from build123d import *

# Parameters (mm, degrees)
EXTRUDE_1_DEPTH     = 40.5
SKETCH_2_R          = 1.75
CUT_EXTRUDE_1_DEPTH = 44
FILLET_6_R          = 5
SKETCH_5_R          = 3
CUT_EXTRUDE_2_DEPTH = 35
SKETCH_6_R          = 7.5
CUT_EXTRUDE_3_DEPTH = 10
CUT_EXTRUDE_4_REACH = 76.382
SKETCH_8_R          = 28.5
SKETCH_4_W          = 7.7
SKETCH_4_H          = 50
CUT_EXTRUDE_5_DEPTH = 30
SKETCH_9_W          = 74.837423064
SKETCH_9_H          = 60.925338007
CUT_EXTRUDE_6_DEPTH = 10
SKETCH_11_W         = 7.7
SKETCH_11_H         = 26
EXTRUDE_2_DEPTH     = 1.5
FILLET_12_R         = 2.5
FILLET_13_R         = 1
FILLET_14_R         = 1
FILLET_15_R         = 2.5
FILLET_START        = 25.8
FILLET_16_DEPTH     = 8.2
FILLET_16_2_ANGLE   = 90
FILLET_17_R         = 1


with BuildPart() as part:
    # 草图1 → 凸台-拉伸1 (new body)
    with BuildSketch(Plane(origin=(0, 0, 0), x_dir=(1, 0, 0), z_dir=(0, 1, 0))):
        with BuildLine():
            Line((0, 28.5), (-22, 28.5))
            Line((-22, 28.5), (-22, -28.5))
            Line((-22, -28.5), (0, -28.5))
            ThreePointArc((0, -28.5), (20.152543264, -20.152543264), (28.5, 0))
            Line((28.5, 0), (28.5, 2.5))
            Line((28.5, 2.5), (33.5, 2.5))
            Line((33.5, 2.5), (33.5, 28.5))
            Line((33.5, 28.5), (0, 28.5))
        make_face()
    extrude(amount=EXTRUDE_1_DEPTH)

    # 草图2 → 切除-拉伸1 (cut)
    with BuildSketch(Plane(origin=(0, 40.5, 0), x_dir=(1, 0, 0), z_dir=(0, 1, 0))):
        with Locations(Location((-13.5, 0, 0), (0, 0, 270))):
            Circle(SKETCH_2_R)
        with Locations(Location((-6.75, 11.691342951, 0), (0, 0, 270))):
            Circle(SKETCH_2_R)
        with Locations(Location((6.75, 11.691342951, 0), (0, 0, 270))):
            Circle(SKETCH_2_R)
        with Locations(Location((13.5, 0, 0), (0, 0, 270))):
            Circle(SKETCH_2_R)
        with Locations(Location((6.75, -11.691342951, 0), (0, 0, 270))):
            Circle(SKETCH_2_R)
        with Locations(Location((-6.75, -11.691342951, 0), (0, 0, 270))):
            Circle(SKETCH_2_R)
    extrude(amount=-CUT_EXTRUDE_1_DEPTH, mode=Mode.SUBTRACT)

    # 圆角6
    fillet_6_edges = [part.edges().sort_by_distance(p)[0] for p in [
        (-22, 20.25, 28.5),
        (-22, 20.25, -28.5),
    ]]
    fillet(fillet_6_edges, radius=FILLET_6_R)

    # 草图5 → 切除-拉伸2 (cut)
    with BuildSketch(Plane(origin=(0, 40.5, 0), x_dir=(1, 0, 0), z_dir=(0, 1, 0))):
        with Locations(Location((-13.5, 0, 0), (0, 0, 270))):
            Circle(SKETCH_5_R)
        with Locations(Location((-6.75, 11.691342951, 0), (0, 0, 270))):
            Circle(SKETCH_5_R)
        with Locations(Location((6.75, 11.691342951, 0), (0, 0, 270))):
            Circle(SKETCH_5_R)
        with Locations(Location((13.5, 0, 0), (0, 0, 270))):
            Circle(SKETCH_5_R)
        with Locations(Location((6.75, -11.691342951, 0), (0, 0, 270))):
            Circle(SKETCH_5_R)
        with Locations(Location((-6.75, -11.691342951, 0), (0, 0, 270))):
            Circle(SKETCH_5_R)
    extrude(amount=-CUT_EXTRUDE_2_DEPTH, mode=Mode.SUBTRACT)

    # 草图6 → 切除-拉伸3 (cut)
    with BuildSketch(Plane(origin=(0, 40.5, 0), x_dir=(1, 0, 0), z_dir=(0, 1, 0))):
        with Locations(Location((0, 0, 0), (0, 0, 270))):
            Circle(SKETCH_6_R)
    extrude(amount=-CUT_EXTRUDE_3_DEPTH, mode=Mode.SUBTRACT)

    # 切除-拉伸4: up to this face of the body (flat: up to its plane)
    cut_extrude_4_end = Plane(part.part.faces().sort_by_distance((28.5, 20.25, -1.25))[0])
    # 草图8 → 切除-拉伸4 (cut, up to the picked face)
    with BuildSketch(Plane.ZY.offset(22), mode=Mode.PRIVATE) as cut_extrude_4_sk1:
        with Locations((0, 40.5)):
            Circle(SKETCH_8_R)
    cut_extrude_4_tool1 = split(extrude(cut_extrude_4_sk1.sketch, amount=-CUT_EXTRUDE_4_REACH, mode=Mode.PRIVATE), bisect_by=cut_extrude_4_end, keep=Keep.BOTH, mode=Mode.PRIVATE)
    add(cut_extrude_4_tool1.solids().sort_by(Axis((-22, 40.5, 0), (1, 0, 0)))[0], mode=Mode.SUBTRACT)

    # 草图4 → 切除-拉伸5 (cut)
    with BuildSketch(Plane(origin=(0, 40.5, 0), x_dir=(1, 0, 0), z_dir=(0, 1, 0))):
        with Locations((29.65, 3.5)):
            Rectangle(SKETCH_4_W, SKETCH_4_H)
    extrude(amount=-CUT_EXTRUDE_5_DEPTH, mode=Mode.SUBTRACT)

    # 草图9 → 切除-拉伸6 (cut)
    with BuildSketch(Plane(origin=(0, 40.5, 0), x_dir=(1, 0, 0), z_dir=(0, 1, 0))):
        with Locations((5.520272929, 0.012240625)):
            Rectangle(SKETCH_9_W, SKETCH_9_H)
    extrude(amount=-CUT_EXTRUDE_6_DEPTH, mode=Mode.SUBTRACT)

    # 草图11 → 凸台-拉伸2 (add)
    with BuildSketch(Plane(origin=(0, 10.5, 0), x_dir=(1, 0, 0), z_dir=(0, 1, 0))):
        with Locations((29.65, 15.5)):
            Rectangle(SKETCH_11_W, SKETCH_11_H)
    extrude(amount=EXTRUDE_2_DEPTH)

    # 圆角12
    fillet_12_edges = [part.edges().sort_by_distance(p)[0] for p in [
        (33.5, 6, -2.5),
        (28.5, 5.25, -2.5),
    ]]
    fillet(fillet_12_edges, radius=FILLET_12_R - 0.0001)  # a hair under: the kernel refuses the full size

    # 圆角13
    fillet_13_edges = [part.edges().sort_by_distance(p)[0] for p in [
        (25.8, 10.5, 4.804130821),
    ]]
    fillet(fillet_13_edges, radius=FILLET_13_R)

    # 圆角14
    fillet_14_edges = [part.edges().sort_by_distance(p)[0] for p in [
        (33.5, 12, -16.74995),
        (32.767796242, 12, -3.232203758),
        (28.40005, 12, -2.5),
    ]]
    fillet(fillet_14_edges, radius=FILLET_14_R)

    # 圆角15
    # the kernel refuses this fillet: 2.5 mm, written as the material it takes off along each edge
    with BuildSketch(Plane(origin=(33.5, 17.25, -28.5), x_dir=(-1, 0, 0), z_dir=(0, -1, 0))) as fillet_15_piece_1:
        with BuildLine():
            CenterArc((FILLET_15_R, -FILLET_15_R), FILLET_15_R, 90, 90)
            Line((0, -FILLET_15_R), (0, 0))
            Line((0, 0), (FILLET_15_R, 0))
        make_face()
    extrude(amount=23.5, mode=Mode.SUBTRACT)

    # 圆角16: read off the stored shape, not the designer's step
    # 圆角16 outline → 圆角16 (cut)
    with BuildSketch(Plane.YZ.offset(FILLET_START)):
        with BuildLine():
            Line((12, -28.5), (12, -27.5))
            ThreePointArc((12, -27.5), (11.707106781, -28.207106781), (11, -28.5))
            Line((11, -28.5), (12, -28.5))
        make_face()
    extrude(amount=FILLET_16_DEPTH, mode=Mode.SUBTRACT)

    # Fillet 16 2 outline → Fillet 16 2 (revolve, cut)
    with BuildSketch(Plane(origin=(31, 0, -26), x_dir=(1, 0, 0), z_dir=(0, 0, 1))):
        with BuildLine():
            Line((2.5, 12), (1.5, 12))
            ThreePointArc((1.5, 12), (2.207106781, 11.707106781), (2.5, 11))
            Line((2.5, 11), (2.5, 12))
        make_face()
    revolve(axis=Axis((31, 0, -26), (0, 1, 0)), revolution_arc=FILLET_16_2_ANGLE, mode=Mode.SUBTRACT)

    # 圆角17
    fillet_17_edges = [part.edges().sort_by_distance(p)[0] for p in [
        (-19.128372458, 30.5, -28.024381801),
        (4.4, 30.5, -28.5),
        (-19.128372458, 30.5, 28.024381801),
        (5.081419572, 30.5, 28.043344578),
        (-8.5, 30.5, 28.5),
    ]]
    fillet(fillet_17_edges, radius=FILLET_17_R)


solid = part.part
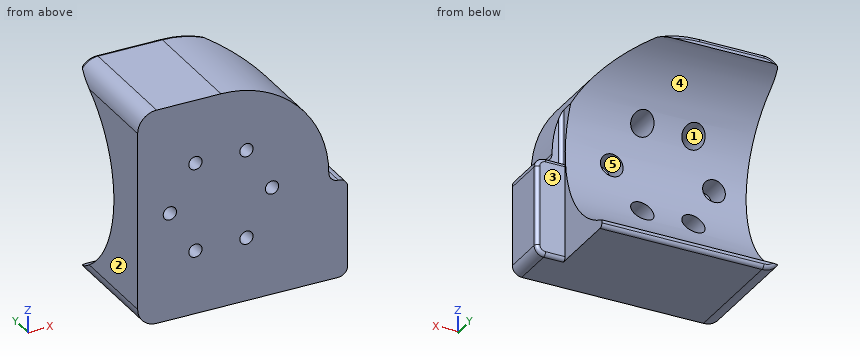
Can you work these out from the model? Positions are in its coordinate system, mm. Face numbers are marked on the shaded views. A direction names the side the tool comes from. Round coordinates to 2 decimals unless told otherwise and drop trailing zeros. Write each loop counter-clockwise with the first axis right and the second up, starting at its lowest first coordinate (ties: lowest second). Pieces come first, ordered by that corner, then holes. Notation, with made-up numbers: M 77,-13.5 L 93,-13.5 A3 cw 93,-8.5 Z; hole C -7,45 d7. An arc over 180 degrees is marked long. Use a Markdown table: item, result.
Item 1: I want a section at D-D (x = -6.75). List the corners of the cut face in (y, z) for me, and give its area (3 significant figures).
Found:
| item | result |
|---|---|
| outline | M 0,-28.5 L 29.5,-28.5 A1 ccw 30.5,-27.5 L 30.5,-26.69 A28.5 cw 16.08,-14.69 L 5.5,-14.69 L 5.5,-13.44 L 0,-13.44 Z; M 0,-9.94 L 5.5,-9.94 L 5.5,-8.69 L 13.36,-8.69 A28.5 cw 13.36,8.69 L 5.5,8.69 L 5.5,9.94 L 0,9.94 Z; M 0,13.44 L 5.5,13.44 L 5.5,14.69 L 16.08,14.69 A28.5 cw 30.5,26.69 L 30.5,27.5 A1 ccw 29.5,28.5 L 0,28.5 Z |
| area | 873 mm2 |
Item 2: Which directions (+Z, -Z, +X, -X, +Y, -Y) give clear straight access to the entire face, cutting with the end or side of a thin tool? Please do the marked faces 4 and 5.
Found:
| item | result |
|---|---|
| face 4 | +X, -X, +Y |
| face 5 | +Y |
Item 3: I want a section at C-C (y = 28.5). List the corners of the cut face in (x, z) for me.
Found:
| item | result |
|---|---|
| outline | M -21.41,-25.85 A5 ccw -17,-28.5 L 25.8,-28.5 L 25.8,-25.85 Z; M -21.41,25.85 L 12,25.85 A28.5 ccw 0,28.5 L -17,28.5 A5 ccw Z |
Item 4: For pin 1 Ø9.5 at (x, z) = (6.75, 11.69) entering from +Y; pin 2 Ø3 at (x, y) = (4, 26.5) entering from +Z; pin 3 Ø5 at (x, z) = (-12.5, 1) entering from +Y, each with a flat end and sliding along its axis, tell me the tip position at first contact or that it passes through.
Found:
| item | result |
|---|---|
| pin 1 | stops at y = 17.22 |
| pin 2 | stops at z = 28.39 |
| pin 3 | stops at y = 12.22 |
Item 5: I want a section at A-A (y = 2). State how many separate pieces and enclosed holes the cut face has, and give its area (3 significant figures).
Found:
| item | result |
|---|---|
| separate pieces | 1 |
| enclosed holes | 6 |
| area | 2,760 mm2 |
Item 6: If I drill on line 1 along Z through (x, y) = (-6.75, 10.75); line 2 along X through (y, z) = (11, 0); line 3 along Z through (x, y) = (-6, 9), over which ranges is the centre line in solid material (lowest first)? Write a range as [from, to].
Found:
| item | result |
|---|---|
| line 1 | z = [-28.5, -14.69], [-8.69, 8.69], [14.69, 28.5] |
| line 2 | x = [-22, -16.5], [-10.5, 10.5], [16.5, 25.93] |
| line 3 | z = [-28.5, -14.6], [-8.79, 8.79], [14.6, 28.5] |
Item 7: I want a section at B-B (x = -13.5). List the corners of the cut face in (y, z) for me.
Found:
| item | result |
|---|---|
| outline | M 0,-28.5 L 29.5,-28.5 A1 ccw 30.5,-27.5 L 30.5,-26.69 A28.5 cw 12.16,-3 L 5.5,-3 L 5.5,-1.75 L 0,-1.75 Z; M 0,1.75 L 5.5,1.75 L 5.5,3 L 12.16,3 A28.5 cw 30.5,26.69 L 30.5,27.5 A1 ccw 29.5,28.5 L 0,28.5 Z |
Item 8: We'd pull the mould along X, two halves only. Please class the marked faces 1, 2 and 3: released by +X, released by -X, zero draft, split by the parting line, or undercut.
Found:
| item | result |
|---|---|
| face 1 | undercut |
| face 2 | released by -X |
| face 3 | zero draft |
